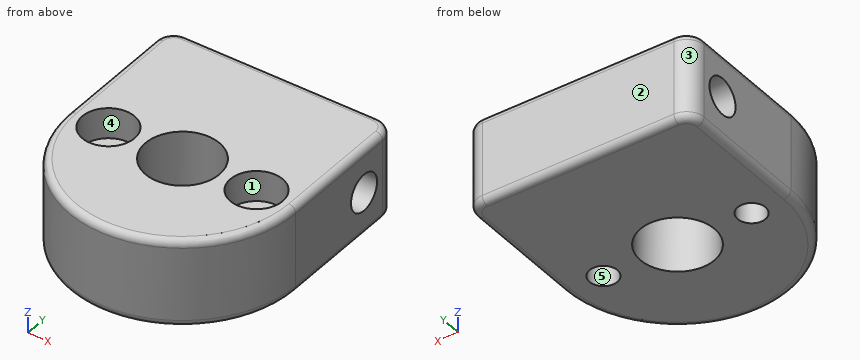
```python
from build123d import *

# Parameters (mm, degrees)
ESQUISSE1_R             = 1.6
ESQUISSE1_R_2           = 4.25
BOSS_EXTRU_1_DEPTH      = 10
ESQUISSE2_R             = 3
ENL_V_MAT_EXTRU_1_DEPTH = 3.5
ESQUISSE3_R             = 2.1
ENL_V_MAT_EXTRU_2_DEPTH = 33.124756808
CONG_1_R                = 2
CONG_2_R                = 0.8


with BuildPart() as part:
    # Esquisse1 → Boss.-Extru.1 (new body)
    with BuildSketch(Plane.XY):
        with BuildLine():
            Line((-13, 16), (13, 16))
            Line((13, 16), (13, 0))
            ThreePointArc((13, 0), (0, -13), (-13, 0))
            Line((-13, 0), (-13, 16))
        make_face()
        with Locations((-8.5, 0)):
            Circle(ESQUISSE1_R, mode=Mode.SUBTRACT)
        with Locations(Location((8.5, 0, 0), (0, 0, 180))):
            Circle(ESQUISSE1_R, mode=Mode.SUBTRACT)
        Circle(ESQUISSE1_R_2, mode=Mode.SUBTRACT)
    extrude(amount=BOSS_EXTRU_1_DEPTH)

    # Esquisse2 → Enlèv. mat.-Extru.1 (cut)
    with BuildSketch(Plane.XY.offset(10)):
        with Locations((-8.5, 0)):
            Circle(ESQUISSE2_R)
        with Locations((8.5, 0)):
            Circle(ESQUISSE2_R)
    extrude(amount=-ENL_V_MAT_EXTRU_1_DEPTH, mode=Mode.SUBTRACT)

    # Esquisse3 → Enlèv. mat.-Extru.2 (cut, through all)
    with BuildSketch(Plane.ZY.offset(13)):
        with Locations(Location((5, 11, 0), (0, 0, 270))):
            Circle(ESQUISSE3_R)
    extrude(amount=-ENL_V_MAT_EXTRU_2_DEPTH, mode=Mode.SUBTRACT)

    # Congé1
    cong_1_edges = [part.edges().sort_by_distance(p)[0] for p in [
        (-13, 16, 5),
        (13, 16, 5),
    ]]
    fillet(cong_1_edges, radius=CONG_1_R)

    # Congé2
    cong_2_edges = [part.edges().sort_by_distance(p)[0] for p in [
        (13, 7, 10),
        (0, 16, 0),
        (0, 16, 10),
        (-13, 7, 0),
        (-12.414213562, 15.414213562, 0),
        (12.414213562, 15.414213562, 0),
        (-13, 7, 10),
        (-12.414213562, 15.414213562, 10),
        (12.414213562, 15.414213562, 10),
        (13, 7, 0),
        (0, -13, 0),
        (0, -13, 10),
    ]]
    fillet(cong_2_edges, radius=CONG_2_R)


solid = part.part
```
Check sheet for the modelled part. Datum: model origin and axes. Units: mm. Face numbers are marked on the shaded views. A direction names the side the tool comes from. Give positions to 0.01 mm unless a question says otherwise; leave off trailing zeros. Write each loop counter-clockwise with the first axis right and the second up, starting at its lowest first coordinate (ties: lowest second). Pieces come first, ordered by that corner, then holes.
Item 1: Cross-section at B-B (x = 0). Enter the section's corners in (y, z).
Item 2: Cross-section at A-A (z = 5). Enter the section's corners in (x, y).
Item 3: Access from +Z, -Z, +X, -X, +Y, -Y to the whole of each face (thin tool, end or side, straight path). Record for the marked faces 4 and 5.
Item 4: Cross-section at D-D (z = 2.5). Enter the section's corners in (x, y).
Item 5: Cross-section at C-C (y = 11). Enter the section's corners in (x, z), and give its area (3 significant figures).
Item 6: Gauge pin test, flat ends, axial feed: pin 1 (6.5 mm diameter, centred on x = 7.5, y = 1, fed in from +Z); pin 2 (3 mm diameter, centred on y = -9, z = 7.5, fed in from +X); pin 3 (5.5 mm diameter, centred on x = 8.5, y = 0, fed in from +Z); pin 4 (5 mm diameter, centred on x = -10.5, z = 5.5, fed in from -Y). Record the tip position at first contact, or that the pin passes through.
Item 7: Scan lines: L1, parallel to Z at x = 6, y = 11; L2, parallel to Y at x = 0, z = 2.5; L3, parallel to X at y = -0.5, z = 4.5. Record each from-to range of solid material in increasing order.
Item 8: Draft check along X on the marked faces 1, 2 and 3. Enter one of: released by +X, released by -X, zero draft, split by the parting line, or undercut.
Report:
1. outline: (-13, 0.8) arc R0.8 ccw to (-12.2, 0) - (-4.25, 0) - (-4.25, 10) - (-12.2, 10) arc R0.8 ccw to (-13, 9.2) - close; (4.25, 0) - (15.2, 0) arc R0.8 ccw to (16, 0.8) - (16, 9.2) arc R0.8 ccw to (15.2, 10) - (4.25, 10) - close; hole circle Ø4.2 at (11, 5)
2. outline: (-13, 0) arc R13 ccw to (13, 0) - (13, 8.9) - (-13, 8.9) - close; (-13, 13.1) - (13, 13.1) - (13, 14) arc R2 ccw to (11, 16) - (-11, 16) arc R2 ccw to (-13, 14) - close; hole circle Ø3.2 at (-8.5, 0); hole circle Ø8.5 at (0, 0); hole circle Ø3.2 at (8.5, 0)
3. face 4: +Z
3. face 5: +Z, -Z
4. outline: (-13, 0) arc R13 ccw to (13, 0) - (13, 14) arc R2 ccw to (11, 16) - (-11, 16) arc R2 ccw to (-13, 14) - close; hole circle Ø3.2 at (-8.5, 0); hole circle Ø8.5 at (0, 0); hole circle Ø3.2 at (8.5, 0)
5. outline: (-13, 0.8) arc R0.8 ccw to (-12.2, 0) - (12.2, 0) arc R0.8 ccw to (13, 0.8) - (13, 2.9) - (-13, 2.9) - close; (-13, 7.1) - (13, 7.1) - (13, 9.2) arc R0.8 ccw to (12.2, 10) - (-12.2, 10) arc R0.8 ccw to (-13, 9.2) - close
5. area: 150 mm2
6. pin 1: stops at z = 10
6. pin 2: stops at x = 10.62
6. pin 3: stops at z = 6.5
6. pin 4: stops at y = -10.25
7. L1: z = 0 to 2.9, 7.1 to 10
7. L2: y = -13 to -4.25, 4.25 to 16
7. L3: x = -12.99 to -10.02, -6.98 to -4.22, 4.22 to 6.98, 10.02 to 12.99
8. face 1: undercut
8. face 2: zero draft
8. face 3: released by -X
